Print and shaded views of the part. All mm, measured from the part's lowest x, y and z. Give positions to 0.01 mm unless a question says otherwise; leave off trailing zeros. Loops run counter-clockwise (first coordinate to the right, second up) from the corner with the lowest first, then second, coordinate; pieces in that order, holes last.
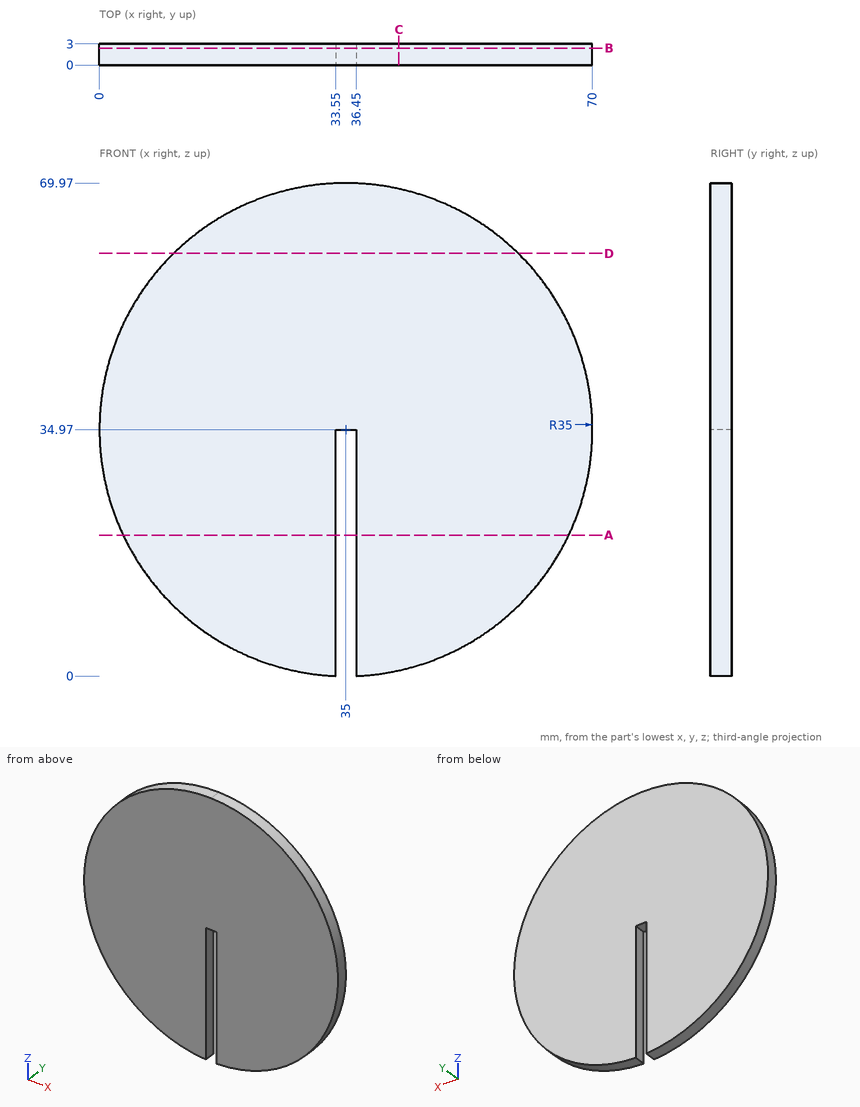
1. Probe line 1 along X through (y, z) = (1.5, 13.5); line 2 along X through (y, z) = (1.25, 16); line 3 along X through (y, z) = (1.6, 53). List the from-to ranges inside material, lowest first.
Responses:
line 1: x = 7.36 to 33.55, 36.45 to 62.64
line 2: x = 5.59 to 33.55, 36.45 to 64.41
line 3: x = 5 to 65
2. Saw through at A-A, the plane z = 20. List the corners of the cut face in (x, y).
Responses:
outline: (3.36, 0) - (33.55, 0) - (33.55, 3) - (3.36, 3) - close; (36.45, 0) - (66.64, 0) - (66.64, 3) - (36.45, 3) - close
3. Saw through at C-C, the plane x = 42.5. List the corners of the cut face in (y, z), and give its area (3 significant figures).
Responses:
outline: (0, 0.78) - (3, 0.78) - (3, 69.16) - (0, 69.16) - close
area: 205 mm2
4. Saw through at B-B, the plane y = 2.4. List the corners of the cut face in (x, z).
Responses:
outline: (33.55, 0) - (33.55, 34.97) - (36.45, 34.97) - (36.45, 0) arc R35 ccw (long way) to start
5. Drop flat-ended pins along their axis: pin 1 (0.9 mm diameter, centred on y = 1.5, z = 15, fed in from +X); pin 2 (1 mm diameter, centred on y = 2, z = 54.5, fed in from -X); pin 3 (0.9 mm diameter, centred on x = 35, y = 1, fed in from -Z). Give the stop position or say it passes through.
Responses:
pin 1: stops at x = 64.05
pin 2: stops at x = 5.63
pin 3: stops at z = 34.97
6. Saw through at D-D, the plane z = 60. List the corners of the cut face in (x, y).
Responses:
outline: (10.54, 0) - (59.46, 0) - (59.46, 3) - (10.54, 3) - close
